Autodesk Inventor part; units mm, degrees
ref_plane "YZ Plane" through (0, 0, 0) normal (1, 0, 0) x (0, 1, 0)
ref_plane "XZ Plane" through (0, 0, 0) normal (0, 1, 0) x (-1, 0, 0)
ref_plane "XY Plane" through (0, 0, 0) normal (0, 0, 1) x (1, 0, 0)
sketch "Sketch1" plane through (0, 0, 0) normal (0, 0, 1) x (1, 0, 0)
  line L0 (-49, 0) -> (49, 0) construction
  line L1 (-53.7631, 0) -> (-51.3816, 4.125)
  line L2 (-51.3816, 4.125) -> (-46.6184, 4.125)
  line L3 (-46.6184, 4.125) -> (-44.2369, 0)
  line L4 (-44.2369, 0) -> (-46.6184, -4.125)
  line L5 (-46.6184, -4.125) -> (-51.3816, -4.125)
  line L6 (-51.3816, -4.125) -> (-53.7631, 0)
  line L7 (53.7631, 0) -> (51.3816, -4.125)
  line L8 (51.3816, -4.125) -> (46.6184, -4.125)
  line L9 (46.6184, -4.125) -> (44.2369, 0)
  line L10 (44.2369, 0) -> (46.6184, 4.125)
  line L11 (46.6184, 4.125) -> (51.3816, 4.125)
  line L12 (51.3816, 4.125) -> (53.7631, 0)
  line L13 (57, -8) -> (-57, -8)
  line L14 (-57, -8) -> (-57, 8)
  line L15 (-57, 8) -> (57, 8)
  line L16 (57, 8) -> (57, -8)
  line L17 (57, -8) -> (-57, 8) construction
  line L18 (-57, -8) -> (57, 8) construction
  line L19 (-57, -6.75) -> (57, -6.75)
  circle A0 centre (-49, 0) radius 8
  circle A1 centre (49, 0) radius 8
  point P0 (0, 0)
  point P1 (0, 0)
  point P2 (49, 8)
  point P3 (-49, 8)
  point P4 (-57, 0)
  point P5 (57, 0)
  dimension "d0" = 98
  dimension "d1" = 8.25
  dimension "d2" = 16
  dimension "d3" = 8
  dimension "d4" = 8
  dimension "d34" = 6.75
extrude "Extrusion1" add sketch "Sketch1" against normal blind 12 contours L1 L2 L3 L4 L5 L6 | L7 L8 L9 L10 L11 L12 | L19 A1 L16 | A1 L19 | L19 A0 L15 A1 | A0 L19 | L19 L14 A0 picked at (48.2061, -5.875) picked at (-49.7939, -5.875)
chamfer "Chamfer2" distance 2 angle 45 5 edges at (0, 8, -12) (54.6569, 5.6569, -12) (57, -3.375, -12) (-54.6569, 5.6569, -12) (-57, -3.375, -12)
sketch "Sketch2" plane through (-49, 8, 0) normal (0, 1, 0) x (1, 0, 0)
  line L0 (11.5, 6) -> (86.5, 6) construction
  line L1 (98, 0) -> (0, 0)
  line L2 (98, 12) -> (0, 12)
  line L3 (49, 0) -> (49, 12) construction
  point P0 (49, 6)
  dimension "d14" = 75
hole "Hole1" at (-37.5, 8, -6) at (37.5, 8, -6) direction (0, -1, 0) diameter 5.4 end through all counterbore diameter 9.5 counterbore depth 5
sketch "Sketch3" plane through (0, 0, 0) normal (0, 0, 1) x (1, 0, 0)
  line L0 (-57, -6.75) -> (57, -6.75)
  arc A0 (-49, 8) -> (-57, 0) centre (-49, 0) ccw
  line L1 (-57, 0) -> (-57, -6.75)
  line L2 (57, -6.75) -> (57, 0)
  arc A1 (57, 0) -> (49, 8) centre (49, 0) ccw
  line L3 (49, 8) -> (-49, 8)
  point P0 (0, 0)
hole "Hole2" at (-49, 0, 0) at (49, 0, 0) direction (0, 0, -1) diameter 6.5 end through all
chamfer "Chamfer3" distance 1 angle 45 2 edges at (-49, 3.25, 0) (49, 3.25, 0)
properties part number "Front Panel Mount" material "ABS Plastic"
Here's how the part is built. I have some questions about the finished solid (model axes, mm). A direction names the side the tool comes from. Coordinates: 2 decimals unless noted, no trailing zeros. Write each loop counter-clockwise with the first axis right and the second up, starting at its lowest first coordinate (ties: lowest second). Pieces come first, ordered by that corner, then holes. Notation, with made-up numbers: (-6, -14.75) -> (50, -14.75) arc R38 ccw to (50, 24.25) -> close; hole circle Ø9 at (62.5, 46). An arc over 180 degrees is marked (long way). Use a Markdown table: item, result. Add a question column.
(1) Please list where these lines run through material, in increasing order: line 1 (Z direction, x = -37.5, y = 4.15); line 2 (X direction, y = 0.5, z = -6); line 3 (Z direction, x = 37.5, y = 0.5).
(2) We'd pull the mould along X, two halves only. Please class faces 1 (the conical face through (53.7, 4.59, -11.43)), 2 (the cylindrical face through (-38.93, 5.47, -1.47)), 3 (the flat face through (-1, 7, -11)): +X half, -X half, draft (parallel to the pull), parting line (faces both ways), or undercut.
(3) If we section it at A-A, the plane x = 37.5: Write out the boundary of the cut face in (y, z).
(4) If we section it at B-B, the plane z = -7.5: Write out the boundary of the cut face in (x, y) (3 decimals), and give its area (3 significant figures).
(5) I'm going to push flat-ended pins straight in: P1, Ø5.5, axis at x = -37.5, z = -6, coming from the -Y side; P2, Ø6, axis at x = 37.5, z = -6, coming from the +Y side; P3, Ø5, axis at y = 4, z = -4.5, coming from the -X side. Where does each tip first touch, or does it pass through?
(6) For faces 4 (the cylindrical face through (39.895, -1.943, -4.754)), 5 (the flat face through (-35, 3, -4)), which set-ups out of +Z, -Z, +X, -X, +Y, -Y let a thin tool reach every point of the face, with its end or its side?
Outcome:
| question | item | result |
|---|---|---|
| 1 | line 1 | z = -12 to -10.75, -1.25 to 0 |
| 1 | line 2 | x = -56.98 to -52.21, -45.79 to -40.2, -34.8 to 34.8, 40.2 to 45.79, 52.21 to 56.98 |
| 1 | line 3 | z = -12 to -8.7, -3.3 to 0 |
| 2 | face 1 | +X half |
| 2 | face 2 | undercut |
| 2 | face 3 | draft |
| 3 | outline | (-6.75, -12) -> (6, -12) -> (7.25, -10.75) -> (3, -10.75) -> (3, -8.7) -> (-6.75, -8.7) -> close; (-6.75, -3.3) -> (3, -3.3) -> (3, -1.25) -> (8, -1.25) -> (8, 0) -> (-6.75, 0) -> close |
| 4 | outline | (-57, -6.75) -> (-39.745, -6.75) -> (-39.745, 3) -> (-42.007, 3) -> (-42.007, 8) -> (-49, 8) arc R8 ccw to (-57, 0) -> close; (-35.255, -6.75) -> (35.255, -6.75) -> (35.255, 3) -> (32.993, 3) -> (32.993, 8) -> (-32.993, 8) -> (-32.993, 3) -> (-35.255, 3) -> close; (39.745, -6.75) -> (57, -6.75) -> (57, 0) arc R8 ccw to (49, 8) -> (42.007, 8) -> (42.007, 3) -> (39.745, 3) -> close; hole circle Ø6.5 at (-49, 0); hole circle Ø6.5 at (49, 0) |
| 4 | area | 1,410 mm^2 |
| 5 | P1 | stops at y = -6.75 |
| 5 | P2 | stops at y = 3 |
| 5 | P3 | stops at x = -56.86 |
| 6 | face 4 | +Y, -Y |
| 6 | face 5 | +Y |
